Geometry check sheet. Reference: drawing and pictorial views, mm from the part's lowest x, y, z. Round coordinates to 2 decimals unless told otherwise and drop trailing zeros. Write each loop counter-clockwise with the first axis right and the second up, starting at its lowest first coordinate (ties: lowest second). Pieces come first, ordered by that corner, then holes. Notation, with made-up numbers: M 45.5,55.5 L 57.5,55.5 A27 cw 57.5,90.5 Z; hole C 5,32.25 d6. An arc over 180 degrees is marked long. Answer in a Markdown table with one row per item.
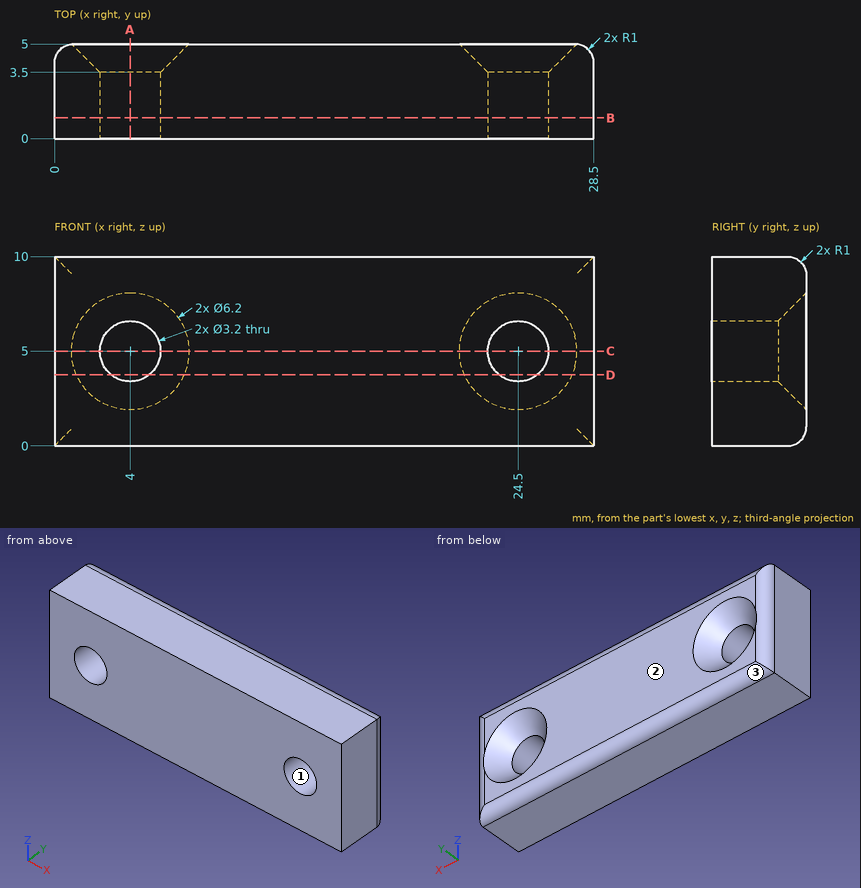
1. Scan lines: L1, parallel to X at y = 1.75, z = 5; L2, parallel to Z at x = 23, y = 4.25; L3, parallel to Z at x = 23.75, y = 0.25. Record each from-to range of solid material in increasing order.
Found:
| item | result |
|---|---|
| L1 | x = 0 to 2.4, 5.6 to 22.9, 26.1 to 28.5 |
| L2 | z = 0.03 to 3.19, 6.81 to 9.97 |
| L3 | z = 0 to 3.59, 6.41 to 10 |
2. Section check D-D, the plane z = 3.75. Count the separate pieces of the cut face and the enclosed holes in it, and give its area (3 significant figures).
Found:
| item | result |
|---|---|
| separate pieces | 3 |
| enclosed holes | 0 |
| area | 116 mm2 |
3. Section check B-B, the plane y = 1.1. Record the cut outline in (x, z).
Found:
| item | result |
|---|---|
| outline | M 0,0 L 28.5,0 L 28.5,10 L 0,10 Z; hole C 4,5 d3.2; hole C 24.5,5 d3.2 |
4. Section check C-C, the plane z = 5. Record the cut outline in (x, y), and give its area (3 significant figures).
Found:
| item | result |
|---|---|
| outline | M 0,0 L 2.4,0 L 2.4,3.5 L 0.9,5 A1 ccw 0,4 Z; M 5.6,0 L 22.9,0 L 22.9,3.5 L 21.4,5 L 7.1,5 L 5.6,3.5 Z; M 26.1,0 L 28.5,0 L 28.5,4 A1 ccw 27.6,5 L 26.1,3.5 Z |
| area | 106 mm2 |
5. Section check A-A, the plane x = 4. Record the cut outline in (y, z).
Found:
| item | result |
|---|---|
| outline | M 0,0 L 4,0 A1 ccw 5,1 L 5,1.9 L 3.5,3.4 L 0,3.4 Z; M 0,6.6 L 3.5,6.6 L 5,8.1 L 5,9 A1 ccw 4,10 L 0,10 Z |
6. Draft check along Z on the marked faces 1, 2 and 3. Enter one of: +Z half, -Z half, draft (parallel to the pull), parting line (faces both ways), or undercut.
Found:
| item | result |
|---|---|
| face 1 | undercut |
| face 2 | draft |
| face 3 | -Z half |
